Input: dimensioned drawing with shaded views. Units: mm. Origin: part minimum x, y, z. Coordinates: 2 decimals unless noted, no trailing zeros. Order: outer loops, then holes, each group sorted by start corner. A loop starts at its lowest first (then second) coordinate and runs counter-clockwise, first axis right, second up. Notation, with made-up numbers: (89.25, 67.5) -> (96.25, 67.5) arc R16 ccw to (96.25, 91.5) -> close; hole circle Ø5 at (21.5, 24.5). An arc over 180 degrees is marked (long way). Put each result on its own line as item: value.
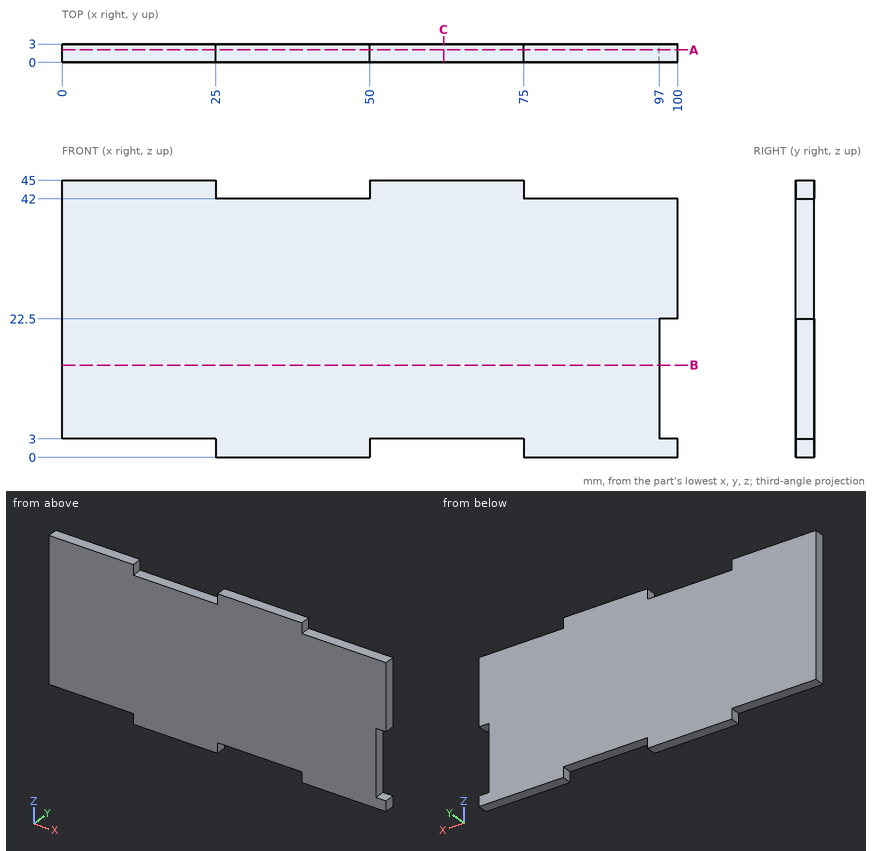
1. Ray query, line 1 along Z through (x, y) = (65, 0.75); line 2 along Z through (x, y) = (92, 0.65); line 3 along X through (y, z) = (2.45, 17). Return the intervals inside material, ascending.
Numbers:
line 1: z = 3 to 45
line 2: z = 0 to 42
line 3: x = 0 to 97
2. Cut plane C-C on x = 62. Output: boundary loops of the cut face in (y, z), plus the area to 3 significant figures.
Numbers:
outline: (0, 3) -> (3, 3) -> (3, 45) -> (0, 45) -> close
area: 126 mm2
3. Cut plane B-B on z = 15. Output: boundary loops of the cut face in (x, y), plus the area to 3 significant figures.
Numbers:
outline: (0, 0) -> (97, 0) -> (97, 3) -> (0, 3) -> close
area: 291 mm2
4. Cut plane A-A on y = 2.05. Output: boundary loops of the cut face in (x, z).
Numbers:
outline: (0, 3) -> (25, 3) -> (25, 0) -> (50, 0) -> (50, 3) -> (75, 3) -> (75, 0) -> (100, 0) -> (100, 3) -> (97, 3) -> (97, 22.5) -> (100, 22.5) -> (100, 42) -> (75, 42) -> (75, 45) -> (50, 45) -> (50, 42) -> (25, 42) -> (25, 45) -> (0, 45) -> close
5. First-contact query: pin 1 (0.9 mm diameter, centred on y = 1, z = 43, fed in from +X); pin 2 (0.9 mm diameter, centred on x = 66.5, y = 1, fed in from -Z); pin 3 (0.9 mm diameter, centred on y = 1.5, z = 10.5, fed in from +X). Flat tips, straight axial feed; report the tip coordinate or a pass-through.
Numbers:
pin 1: stops at x = 75
pin 2: stops at z = 3
pin 3: stops at x = 97
